Can you work these out from the drawing? Everything is in mm from the part's minimum corner. A direction names the side the tool comes from. Give positions to 0.01 mm unless a question says otherwise; leave off trailing zeros. Write each loop counter-clockwise with the first axis right and the second up, starting at its lowest first coordinate (ties: lowest second). Pieces come first, ordered by that corner, then holes. Notation, with made-up numbers: (76, 65) - (106, 65) arc R22 cw to (106, 76) - close; hole circle Ø6 at (-11, -8). An arc over 180 degrees is marked (long way). Answer in a Markdown table with one row per item.
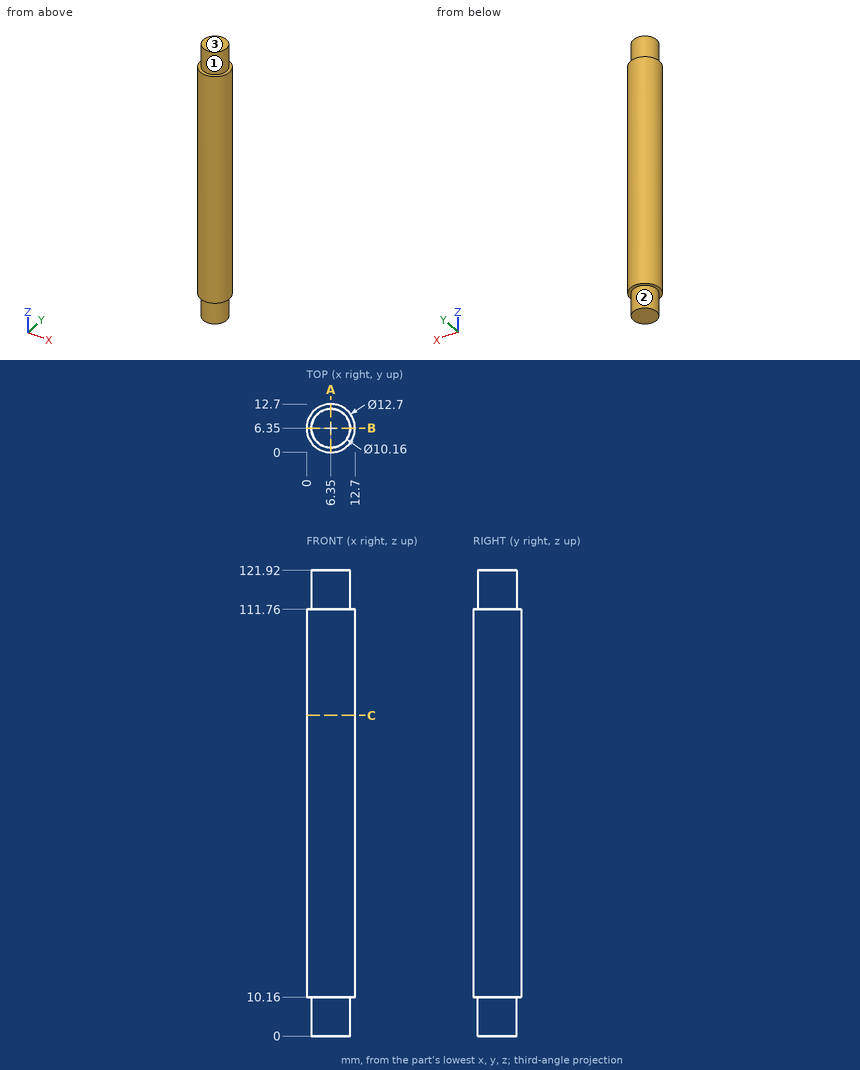
1) Imagine slicing it at C-C (z = 84). List the corners of the cut face in (x, y) for me, then the cut area to 3 significant figures.
Check values:
| item | result |
|---|---|
| outline | circle Ø12.7 at (6.35, 6.35) |
| area | 127 mm2 |
2) If I drill on line 1 (Z direction, x = 9.25, y = 11); line 2 (Y direction, x = 6.5, z = 71); line 3 (X direction, y = 6, z = 59.5), over which ranges is the centre line in solid material (lowest first)?
Check values:
| item | result |
|---|---|
| line 1 | z = 10.16 to 111.76 |
| line 2 | y = 0 to 12.7 |
| line 3 | x = 0.01 to 12.69 |
3) Will these pins go through, and if not, where does the flat tip stop? P1, Ø4, axis at y = 9, z = 87, coming from the +X side; P2, Ø1.5, axis at x = 4, z = 94, coming from the +Y side; P3, Ø6, axis at y = 2, z = 96, coming from the +X side.
Check values:
| item | result |
|---|---|
| P1 | stops at x = 12.67 |
| P2 | stops at y = 12.5 |
| P3 | stops at x = 12.55 |
4) Imagine slicing it at A-A (x = 6.35). List the corners of the cut face in (y, z) for me.
Check values:
| item | result |
|---|---|
| outline | (0, 10.16) - (1.27, 10.16) - (1.27, 0) - (11.43, 0) - (11.43, 10.16) - (12.7, 10.16) - (12.7, 111.76) - (11.43, 111.76) - (11.43, 121.92) - (1.27, 121.92) - (1.27, 111.76) - (0, 111.76) - close |
5) On a 3-axis mill with a long thin cutter (end or side, diameter ignored), from which of +Z, -Z, +X, -X, +Y, -Y can I reach the whole of each face in a straight line? I mean the marked faces 1, 2 and 3. Say none if no direction works.
Check values:
| item | result |
|---|---|
| face 1 | +Z |
| face 2 | -Z |
| face 3 | +Z, +X, -X, +Y, -Y |
